```python
from build123d import *

# Parameters (mm, degrees)
SKETCH_1_W      = 6
SKETCH_1_H      = 3
EXTRUDE_1_DEPTH = 4
EXTRUDE_2_DEPTH = 1


with BuildPart() as part:
    # 草图1 → 凸台-拉伸1 (new body)
    with BuildSketch(Plane.XY):
        with Locations((3, -1.5)):
            Rectangle(SKETCH_1_W, SKETCH_1_H)
    extrude(amount=EXTRUDE_1_DEPTH)

    # 草图2 → 凸台-拉伸2 (add, symmetric)
    with BuildSketch(Plane.XY.offset(2)):
        Polygon((0, -0.453225327), (-0.392993769, -0.453225327), (-1.262945453, -2.502630735), (-1.725619725, -2.502630735), (-1.958016745, -2.979922814), (-1.262945453, -2.979922814), (-0.92927242, -2.979922814), (-0.196496885, -0.979190926), (0, -0.979190926), align=None)
        Polygon((7.725619725, -2.502630735), (7.958016745, -2.979922814), (7.262945453, -2.979922814), (6.92927242, -2.979922814), (6.196496885, -0.979190926), (6, -0.979190926), (6, -0.453225327), (6.392993769, -0.453225327), (7.262945453, -2.502630735), align=None)
    extrude(amount=EXTRUDE_2_DEPTH, both=True)


solid = part.part
```
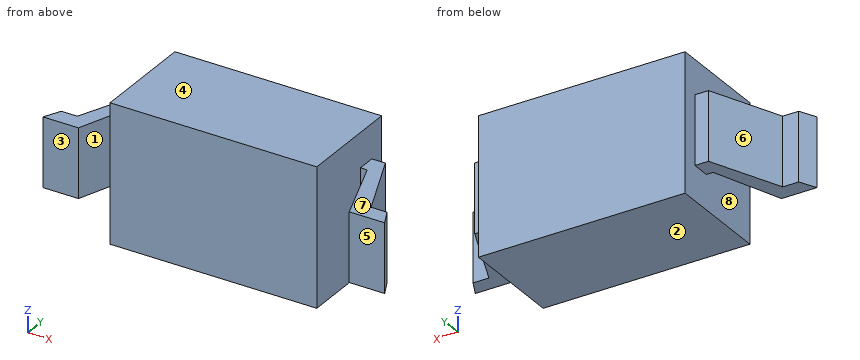
The model under review builds one solid part; all positions refer to its coordinate system, in mm. Face numbers are marked on the shaded views. A direction names the side the tool comes from. Give positions to 0.01 mm unless a question says otherwise; leave off trailing zeros. Write each loop counter-clockwise with the first axis right and the second up, starting at its lowest first coordinate (ties: lowest second). Pieces come first, ordered by that corner, then holes. Notation, with made-up numbers: (-35.75, -38.5) -> (-23.75, -38.5) arc R27 ccw to (-23.75, 0.5) -> close; hole circle Ø2 at (28, -17.75). An arc over 180 degrees is marked (long way). Put each result on its own line as item: value.
(1) We need section A-A, the plane y = -1.2. Give the boundary of the cut face in (x, z).
Results are:
outline: (-0.71, 1) -> (-0.28, 1) -> (-0.28, 3) -> (-0.71, 3) -> close; (0, 0) -> (6, 0) -> (6, 4) -> (0, 4) -> close; (6.28, 1) -> (6.71, 1) -> (6.71, 3) -> (6.28, 3) -> close
(2) We need section C-C, the plane y = -2.75. Give the boundary of the cut face in (x, z), and give its area (3 significant figures).
Results are:
outline: (-1.85, 1) -> (-0.85, 1) -> (-0.85, 3) -> (-1.85, 3) -> close; (0, 0) -> (6, 0) -> (6, 4) -> (0, 4) -> close; (6.85, 1) -> (7.85, 1) -> (7.85, 3) -> (6.85, 3) -> close
area: 28.0 mm²
(3) We need section B-B, the plane z = 2.75. Give the boundary of the cut face in (x, y).
Results are:
outline: (-1.96, -2.98) -> (-0.93, -2.98) -> (-0.2, -0.98) -> (0, -0.98) -> (0, -3) -> (6, -3) -> (6, -0.98) -> (6.2, -0.98) -> (6.93, -2.98) -> (7.96, -2.98) -> (7.73, -2.5) -> (7.26, -2.5) -> (6.39, -0.45) -> (6, -0.45) -> (6, 0) -> (0, 0) -> (0, -0.45) -> (-0.39, -0.45) -> (-1.26, -2.5) -> (-1.73, -2.5) -> close
(4) The part is to be moulded in two halves that separate along X. For the marked faces 6, 7 and 8, say which applies: pulls with the +X half, pulls with the -X half, needs draft (parallel to the pull), parting line crosses it, or undercut.
Results are:
face 6: pulls with the -X half
face 7: needs draft
face 8: undercut
(5) Tool access review of the marked faces 1, 2, 3, 4 and 5: name each direction out of +Z, -Z, +X, -X, +Y, -Y from which nothing blocks a thin tool from reaching the whole face with its end or side.
Results are:
face 1: +Z, -Z, -Y
face 2: -Z, +X, -X, +Y, -Y
face 3: +Z, -Z, -X, -Y
face 4: +Z, +X, -X, +Y, -Y
face 5: +Z, -Z, +X, -Y
(6) We need section D-D, the plane z = 3.6. Give the boundary of the cut face in (x, y).
Results are:
outline: (0, -3) -> (6, -3) -> (6, 0) -> (0, 0) -> close
(7) For pin 1 Ø1 at (y, z) = (-0.5, 1) entering from -X; pin 2 Ø1.6 at (x, y) = (7, -1.5) entering from +Z; pin 3 Ø0.8 at (x, z) = (7.5, 1.5) entering from -Y; pin 4 Ø1 at (x, z) = (1.5, 3) entering from +Y, all flat-tipped, find the tip position at first contact; note any pin that passes through.
Results are:
pin 1: x = -0.63
pin 2: z = 3
pin 3: y = -2.98
pin 4: y = 0
(8) To check wall thickness, follow probe 1 along X at (y, z) = (-2.4, 1.45); probe 2 along X at (y, z) = (-1.7, 2.8); probe 3 along X at (y, z) = (-1.4, 0.9). State the ranges of each line that lie inside material, in increasing order. Write a range as from..to.
Results are:
probe 1: -1.22..-0.72, 0..6, 6.72..7.22
probe 2: -0.92..-0.46, 0..6, 6.46..6.92
probe 3: 0..6
